from build123d import *

# Parameters (mm, degrees)
F1_DEPTH = 16
F2_DEPTH = 1
F3_DEPTH = 2
F4_W     = 3.5
F4_H     = 2
F5_DEPTH = 2.5


with BuildPart() as f1:
    # F0 (on Top) → F1 (new body)
    with BuildSketch(Plane.XY):
        Polygon((5.312592, -1.423505), (0, 0), (-0.776457, -2.897777), (0.189469, -3.156597), (0.707107, -1.224745), (4.087847, -2.130612), (3.570209, -4.062463), (4.536135, -4.321282), (5.158121, -2), align=None)
        Polygon((-2.139903, -11.849929), (-3.105829, -11.59111), (-3.882286, -14.488887), (1.430306, -15.912392), (2.206764, -13.014615), (1.240838, -12.755796), (0.7232, -14.687647), (-2.657541, -13.781781), align=None)
        Polygon((0.189469, -3.156597), (-0.776457, -2.897777), (-3.105829, -11.59111), (-2.139903, -11.849929), align=None)
        Polygon((12, 0), (0, 0), (5.312592, -1.423505), (5.158121, -2), (12, -2), align=None)
    extrude(amount=F1_DEPTH)

    # F0 (on Top) → F2 (join)
    with BuildSketch(Plane.XY):
        Polygon((0.707107, -1.224745), (0.189469, -3.156597), (-2.139903, -11.849929), (-2.657541, -13.781781), (0.7232, -14.687647), (1.240838, -12.755796), (3.570209, -4.062463), (4.087847, -2.130612), align=None)
    extrude(amount=F2_DEPTH)

    # F0 (on Top) → F3 (join)
    with BuildSketch(Plane.XY):
        Polygon((2.206764, -13.014615), (4.536135, -4.321282), (3.570209, -4.062463), (1.240838, -12.755796), align=None)
    extrude(amount=F3_DEPTH)


with BuildPart() as f5:
    # F4 (on Front) → F5 (new body, symmetric)
    with BuildSketch(Plane.XZ):
        with Locations((16.25, 11.703817)):
            Rectangle(F4_W, F4_H)
        with Locations((16.25, 3.703817)):
            Rectangle(F4_W, F4_H)
    extrude(amount=F5_DEPTH, both=True)


with BuildPart() as f5_1:
    # F6: moved
    add(f5.part.moved(Location((-7.5, 0, 0))))


with BuildPart() as f1_1:
    add(f1.part)

    # F7: cut F5
    add(f5_1.part, mode=Mode.SUBTRACT)


solid = f1_1.part
Geometry check sheet. Reference: the model listing, model coordinates, mm. A direction names the side the tool comes from. Give positions to 0.01 mm unless a question says otherwise; leave off trailing zeros. Order: outer loops, then holes, each group sorted by start corner. A loop starts at its lowest first (then second) coordinate and runs counter-clockwise, first axis right, second up.
1) Cross-section at D-D (x = -1.75). Record the boundary of the cut face in (y, z), then the cut area to 3 significant figures.
Results are:
outline: (-15.06, 0) - (-6.53, 0) - (-6.53, 16) - (-10.39, 16) - (-10.39, 1) - (-14.02, 1) - (-14.02, 16) - (-15.06, 16) - close
area: 82.0 mm2
2) Gauge pin test, flat ends, axial feed: pin 1 (2 mm diameter, centred on x = 5, y = -5, fed in from +Z); pin 2 (1.5 mm diameter, centred on y = -13.5, z = 8, fed in from -X); pin 3 (1.6 mm diameter, centred on y = -1, z = 3.5, fed in from -X); pin 4 (3.5 mm diameter, centred on x = 8, z = 9, fed in from -Y). Record the tip position at first contact, or that the pin passes through.
Results are:
pin 1: stops at z = 16
pin 2: stops at x = -3.82
pin 3: stops at x = -0.48
pin 4: stops at y = -2
3) Tool access check on faces 5 (the flat face through (10.5, -1, 12)), 6 (the flat face through (2.37, -1.67, 8.4)), 7 (the flat face through (4.05, -4.19, 8.9)), 8 (the flat face through (9, -2, 8)). Record the directions out of +Z, -Z, +X, -X, +Y, -Y that give a thin tool (end or side, any length) a straight path to the whole face; none if there is none.
Results are:
face 5: +Y, -Y
face 6: +Z
face 7: +Z, -Y
face 8: +Z, -Z, +X, -Y
4) Material ranges on probe 1 along Y at (x, z) = (6.5, 9.75); probe 2 along Z at (x, y) = (0.5, -5); probe 3 along X at (y, z) = (-8, 5.25), recorded low to high.
Results are:
probe 1: y = -2 to 0
probe 2: z = 0 to 1
probe 3: x = -2.14 to -1.11
5) Cross-section at A-A (x = 9.75). Record the boundary of the cut face in (y, z), then the cut area to 3 significant figures.
Results are:
outline: (-2, 0) - (0, 0) - (0, 2.7) - (-2, 2.7) - close; (-2, 4.7) - (0, 4.7) - (0, 10.7) - (-2, 10.7) - close; (-2, 12.7) - (0, 12.7) - (0, 16) - (-2, 16) - close
area: 24.0 mm2
6) Draft check along X on faces 1 (the flat face through (6, 0, 8)), 2 (the flat face through (1, -8, 1)), 3 (the flat face through (9, -1, 12.704)), 4 (the flat face through (1.731, -12.887, 8.902)). Enter one of: released by +X, released by -X, zero draft, split by the parting line, or undercut.
Results are:
face 1: zero draft
face 2: undercut
face 3: undercut
face 4: released by +X
7) Cross-section at C-C (y = -3.5). Record the boundary of the cut face in (x, z), then the cut area to 3 significant figures.
Results are:
outline: (-0.94, 0) - (4.76, 0) - (4.76, 16) - (3.72, 16) - (3.72, 1) - (0.1, 1) - (0.1, 16) - (-0.94, 16) - close
area: 36.8 mm2
8) Cross-section at B-B (z = 11.75). Record the boundary of the cut face in (x, y), then the cut area to 3 significant figures.
Results are:
outline: (-3.88, -14.49) - (1.43, -15.91) - (2.21, -13.01) - (1.24, -12.76) - (0.72, -14.69) - (-2.66, -13.78) - (-2.14, -11.85) - (0.19, -3.16) - (0.71, -1.22) - (4.09, -2.13) - (3.57, -4.06) - (4.54, -4.32) - (5.16, -2) - (7, -2) - (7, 0) - (0, 0) - close; (10.5, -2) - (12, -2) - (12, 0) - (10.5, 0) - close
area: 38.2 mm2
